Build history of the part. All positions in model axes, mm. Face numbers are marked on the shaded views. A direction names the side the tool comes from. Round coordinates to 2 decimals unless told otherwise and drop trailing zeros. Order: outer loops, then holes, each group sorted by start corner. A loop starts at its lowest first (then second) coordinate and runs counter-clockwise, first axis right, second up. Notation, with made-up numbers: M -20.75,72 L 24.25,72 A8 cw 24.25,87 Z; hole C 42.5,5.5 d10. An arc over 180 degrees is marked long. Use CSV: the item, a comma, the result in double quotes.
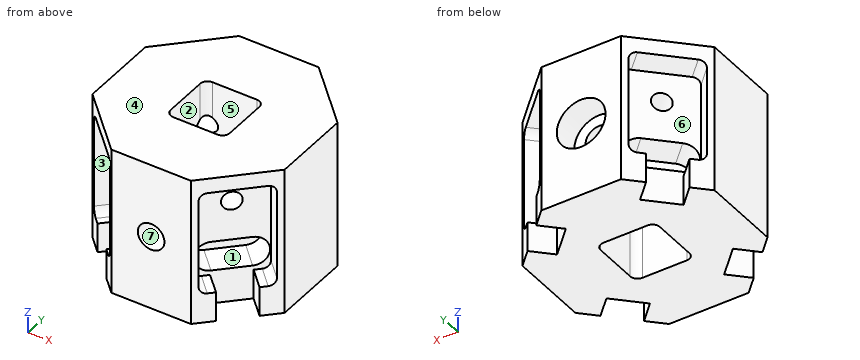
from build123d import *

# Parameters (mm, degrees)
SKETCH1_W                                            = 4
SKETCH1_H                                            = 4
BOSS_EXTRUDE1_DEPTH                                  = 10
FILLET2_R                                            = 0.5
SKETCH11_W                                           = 7
SKETCH11_H                                           = 1
SKETCH11_H_2                                         = 1.25
SKETCH11_W_2                                         = 2
CUT_EXTRUDE3_DEPTH                                   = 1.7
FILLET3_R                                            = 0.5
CUT_EXTRUDE4_DEPTH                                   = 2
CIRPATTERN14_COUNT                                   = 4
FILLET3_OF_CIRPATTERN14_R                            = 0.5
CBORE_FOR_M1_6_HEXAGON_SOCKET_HEAD_CAP_S_D           = 1.8
CBORE_FOR_M1_6_HEXAGON_SOCKET_HEAD_CAP_S_CBORE_D     = 3.3
CBORE_FOR_M1_6_HEXAGON_SOCKET_HEAD_CAP_S_CBORE_DEPTH = 1.8


with BuildPart() as part:
    # Sketch1 → Boss-Extrude1 (new body)
    with BuildSketch(Plane.XY):
        Polygon((-2.692388155, 6.5), (-6.5, 2.692388155), (-6.5, -2.692388155), (-2.692388155, -6.5), (2.692388155, -6.5), (6.5, -2.692388155), (6.5, 2.692388155), (2.692388155, 6.5), align=None)
        Rectangle(SKETCH1_W, SKETCH1_H, mode=Mode.SUBTRACT)
    extrude(amount=BOSS_EXTRUDE1_DEPTH)

    # Fillet2
    fillet2_edges = [part.edges().sort_by_distance(p)[0] for p in [
        (2, -2, 5),
        (2, 2, 5),
        (-2, 2, 5),
        (-2, -2, 5),
    ]]
    fillet(fillet2_edges, radius=FILLET2_R)

    # Sketch11 → Cut-Extrude3 (cut)
    with BuildSketch(Plane(origin=(4.596194078, 4.596194078, 0), x_dir=(0, 0, -1), z_dir=(0.7071067811865477, 0.7071067811865475, 0))):
        with Locations((-5.5, 1.75)):
            Rectangle(SKETCH11_W, SKETCH11_H)
        with Locations((-5.5, 0.625)):
            Rectangle(SKETCH11_W, SKETCH11_H_2)
        with Locations((-5.5, -0.625)):
            Rectangle(SKETCH11_W, SKETCH11_H_2)
        with Locations((-5.5, -1.75)):
            Rectangle(SKETCH11_W, SKETCH11_H)
        with Locations((-1, 0.625)):
            Rectangle(SKETCH11_W_2, SKETCH11_H_2)
        with Locations((-1, -0.625)):
            Rectangle(SKETCH11_W_2, SKETCH11_H_2)
    cut_extrude3 = extrude(amount=-CUT_EXTRUDE3_DEPTH, mode=Mode.SUBTRACT)

    # Fillet3
    fillet3_edges = [part.edges().sort_by_distance(p)[0] for p in [
        (5.586143571, 2.404163056, 9),
        (2.404163056, 5.586143571, 9),
        (2.404163056, 5.586143571, 2),
        (5.586143571, 2.404163056, 2),
    ]]
    fillet(fillet3_edges, radius=FILLET3_R)

    # Sketch13 → Tap Drill for M1.6 Tap2 (revolve, cut)
    with BuildSketch(Plane(origin=(3.39411255, 3.39411255, 7), x_dir=(-0.7071067811865475, 0.7071067811865477, 0), z_dir=(0, 0, 1))):
        Polygon((0, 0), (0, 5.375537887), (0.625, 5), (0.625, 0), align=None)
    tap_drill_for_m1_6_tap2 = revolve(axis=Axis((7.88424061, 7.88424061, 7), (-0.7071067811865477, -0.7071067811865475, 0)), mode=Mode.SUBTRACT)

    # Sketch14 → Cut-Extrude4 (cut)
    with BuildSketch(Plane(origin=(3.39411255, 3.39411255, 0), x_dir=(0, 0, -1), z_dir=(0.7071067811865476, 0.7071067811865476, 0))):
        with BuildLine():
            Line((-2.3, 1.2), (-2.3, -1.2))
            ThreePointArc((-2.3, -1.2), (-3.3, -2.2), (-4.3, -1.2))
            Line((-4.3, -1.2), (-4.3, 1.2))
            ThreePointArc((-4.3, 1.2), (-3.3, 2.2), (-2.3, 1.2))
        make_face()
    cut_extrude4 = extrude(amount=-CUT_EXTRUDE4_DEPTH, mode=Mode.SUBTRACT)

    # CirPattern14: Cut-Extrude3, Tap Drill for M1.6 Tap2, Cut-Extrude4 ×4 about axis
    cirpattern14_axis = Axis((0, 0, 0), (0, 0, 1))
    add([cut_extrude3.rotate(cirpattern14_axis, i * 360 / CIRPATTERN14_COUNT) for i in range(1, CIRPATTERN14_COUNT)], mode=Mode.SUBTRACT)
    add([tap_drill_for_m1_6_tap2.rotate(cirpattern14_axis, i * 360 / CIRPATTERN14_COUNT) for i in range(1, CIRPATTERN14_COUNT)], mode=Mode.SUBTRACT)
    add([cut_extrude4.rotate(cirpattern14_axis, i * 360 / CIRPATTERN14_COUNT) for i in range(1, CIRPATTERN14_COUNT)], mode=Mode.SUBTRACT)

    # Fillet3 of CirPattern14
    fillet3_of_cirpattern14_edges = [part.edges().sort_by_distance(p)[0] for p in [
        (-2.404163056, 5.586143571, 9),
        (-5.586143571, 2.404163056, 9),
        (-5.586143571, 2.404163056, 2),
        (-2.404163056, 5.586143571, 2),
        (-5.586143571, -2.404163056, 9),
        (-2.404163056, -5.586143571, 9),
        (-2.404163056, -5.586143571, 2),
        (-5.586143571, -2.404163056, 2),
        (2.404163056, -5.586143571, 9),
        (5.586143571, -2.404163056, 9),
        (5.586143571, -2.404163056, 2),
        (2.404163056, -5.586143571, 2),
    ]]
    fillet(fillet3_of_cirpattern14_edges, radius=FILLET3_OF_CIRPATTERN14_R)

    # CBORE for M1.6 Hexagon socket head cap s (through all)
    with Locations(Plane(origin=(0, 6.5, 5), x_dir=(0, 0, 1), z_dir=(0, 1, 0))):
        with Locations((0, 0)):
            CounterBoreHole(CBORE_FOR_M1_6_HEXAGON_SOCKET_HEAD_CAP_S_D / 2, CBORE_FOR_M1_6_HEXAGON_SOCKET_HEAD_CAP_S_CBORE_D / 2, CBORE_FOR_M1_6_HEXAGON_SOCKET_HEAD_CAP_S_CBORE_DEPTH)


solid = part.part
(1) Cut at B-B, the plane x = 0. Give the cut face in (y, z).
Answer block:
outline,"M -6.5,0 L -2,0 L -2,4.1 L -6.5,4.1 Z; M -6.5,5.9 L -2,5.9 L -2,10 L -6.5,10 Z; M 2,0 L 6.5,0 L 6.5,3.35 L 4.7,3.35 L 4.7,4.1 L 2,4.1 Z; M 2,5.9 L 4.7,5.9 L 4.7,6.65 L 6.5,6.65 L 6.5,10 L 2,10 Z"
(2) Two-plate mould, pull along Z, no slides. Class the marked faces 4, 5, 6 and 7: released by +Z, released by -Z, zero draft, split by the parting line, or undercut.
Answer block:
face 4,"released by +Z"
face 5,"zero draft"
face 6,"undercut"
face 7,"undercut"
(3) Tool access for the marked faces 1, 2 and 3: list every direction of +Z, -Z, +X, -X, +Y, -Y with a clear straight run to the whole face (end or side of a thin tool).
Answer block:
face 1,"none"
face 2,"+Z, -Z"
face 3,"-Y"
(4) Drop a flat-ended pin along its axis: pin 1 (2.5 mm diameter, centred on x = 0, z = 5, fed in from +Y). Give the stop position or say it passes through.
Answer block:
pin 1,"stops at y = 4.7"
(5) Wall check: line 1 (Y direction, x = 1, z = 4); line 2 (Y direction, x = 0, z = 2.5); line 3 (Z direction, x = 3.5, y = 2.5). Give the ranges that are in metal, low to high. Write a range as from..to.
Answer block:
line 1,"y = -6.5..-3.71, -2.96..-2, 2..2.96, 3.71..4.7"
line 2,"y = -6.5..-2, 2..6.5"
line 3,"z = 0..2.3, 4.3..10"
(6) Cut at A-A, the plane y = 0. Give the cut face in (x, z).
Answer block:
outline,"M -6.5,0 L -2,0 L -2,10 L -6.5,10 Z; M 2,0 L 6.5,0 L 6.5,10 L 2,10 Z"
